Autodesk Inventor part; units mm, degrees
ref_plane "YZ Plane" through (0, 0, 0) normal (1, 0, 0) x (0, 1, 0)
ref_plane "XZ Plane" through (0, 0, 0) normal (0, 1, 0) x (-1, 0, 0)
ref_plane "XY Plane" through (0, 0, 0) normal (0, 0, 1) x (1, 0, 0)
sketch "Sketch1" plane through (0, 0, 0) normal (0, 1, 0) x (-1, 0, 0)
  line L0 (0, 0) -> (71, 0)
  line L1 (71, 0) -> (71, -96)
  line L2 (71, -96) -> (0, -96)
  line L3 (0, -96) -> (0, 0)
  dimension "d0" = 96
  dimension "d1" = 71
extrude "Extrusion1" add sketch "Sketch1" along normal blind 36
sketch "Sketch2" plane through (0, 0, 0) normal (1, 0, 0) x (0, 0, -1)
  line L0 (96, 0) -> (0, 0)
  line L1 (0, 0) -> (0, 23.3)
  line L2 (0, 0) -> (0, 36)
  line L3 (96, 0) -> (96, 36)
  line L4 (0, 23.3) -> (96, 23.3)
  line L5 (96, 23.3) -> (96, 27.8)
  line L6 (96, 27.8) -> (0, 27.8)
  line L7 (0, 27.8) -> (0, 23.3)
  line L8 (6.5, 27.8) -> (89.5, 27.8)
  line L9 (89.5, 27.8) -> (89.5, 23.3)
  line L10 (89.5, 23.3) -> (6.5, 23.3)
  line L11 (6.5, 23.3) -> (6.5, 27.8)
  point P0 (6.5, 23.3)
  point P1 (0, 27.8)
  dimension "d4" = 23.3
  dimension "d5" = 4.5
  dimension "d6" = 83
  dimension "d7" = 6.5
extrude "Extrusion2" cut sketch "Sketch2" against normal blind 112.75 contours L4 L9 L6 L3 | L2 L6 L11 L4
properties part number "Placeholde_stepperdriverr"
Check sheet for the modelled part. Datum: model origin and axes. Units: mm. A direction names the side the tool comes from. Coordinates: 2 decimals unless noted, no trailing zeros. Order: outer loops, then holes, each group sorted by start corner. A loop starts at its lowest first (then second) coordinate and runs counter-clockwise, first axis right, second up. Notation, with made-up numbers: (9.5, 64.5) -> (45.5, 64.5) arc R19 cw to (45.5, 81.5) -> close; hole circle Ø7 at (47, -34.75). An arc over 180 degrees is marked (long way). Write item = value, one per line. Start each with the question number.
1) Material ranges on L1, parallel to Y at x = -50, z = -91.5, recorded low to high.
2) Cross-section at A-A (x = -48.5). Enter the section's corners in (y, z).
3) Access from +Z, -Z, +X, -X, +Y, -Y to the whole of each face (thin tool, end or side, straight path). Record for faces 1 (the flat face through (-35, 11, 0)), 2 (the flat face through (-35, 27.8, -3)), 3 (the flat face through (-35, 23.3, -93)).
4) Go/stop test with flat-tipped pins: P1, Ø1.5, axis at x = -40, y = 26, coming from the +Z side; P2, Ø3.5, axis at x = -18.5, y = 25.5, coming from the -Z side. Record where each tip stops, or that it passes through.
5) Cross-section at B-B (y = 26.5). Enter the section's corners in (x, z), then the cut area to 3 significant figures.
Ans:
q1.L1 = 0 to 23.3, 27.8 to 36
q2.outline = (0, -96) -> (23.3, -96) -> (23.3, -89.5) -> (27.8, -89.5) -> (27.8, -96) -> (36, -96) -> (36, 0) -> (27.8, 0) -> (27.8, -6.5) -> (23.3, -6.5) -> (23.3, 0) -> (0, 0) -> close
q3.face_1 = +Z, +X, -X, +Y, -Y
q3.face_2 = +Z, +X, -X
q3.face_3 = -Z, +X, -X
q4.P1 = -6.5
q4.P2 = -89.5
q5.outline = (-71, -89.5) -> (0, -89.5) -> (0, -6.5) -> (-71, -6.5) -> close
q5.area = 5,890 mm²
